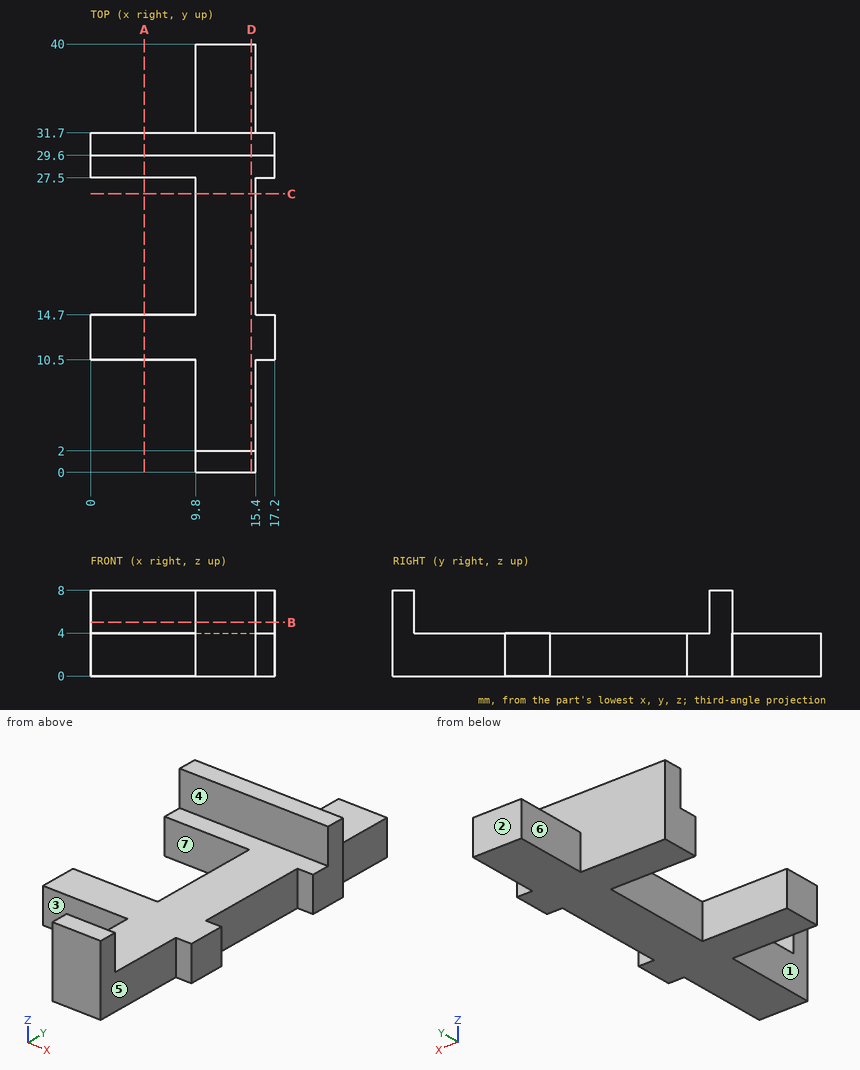
Study the drawing (mm; zero at the part's minimum x, y, z) and answer. A direction names the side the tool comes from. Give positions to 0.01 mm unless a question says otherwise; leave off trailing zeros. Order: outer loops, then holes, each group sorted by start corner. A loop starts at its lowest first (then second) coordinate and runs counter-clockwise, first axis right, second up. Notation, with made-up numbers: (82.25, -28.75) - (107.25, -28.75) arc R11 ccw to (107.25, -18.75) - close; hole circle Ø5 at (73.25, 17). An arc over 180 degrees is marked (long way). Use one line per item in the form item = value. Start each with the question number.
(1) Consider line 1 (Y direction, x = 10, z = 7.75); line 2 (Y direction, x = 4.75, z = 1.5); line 3 (Y direction, x = 9, z = 5.75). Determine where each line is inside the solid, lowest interval first. Write a range as from..to.
(2) A cutting plane is placed at B-B, the plane z = 5. Write down the section's boundary in (x, y).
(3) A cutting plane is placed at C-C, the plane y = 26. Write down the section's boundary in (x, z), then the cut area to 3 significant figures.
(4) A cutting plane is placed at D-D, the plane x = 15. Write down the section's boundary in (y, z).
(5) A cutting plane is placed at A-A, the plane x = 5. Write down the section's boundary in (y, z).
(6) Flat-ended cylindrical pins translate along their axes: pin 1 Ø1 at (y, z) = (22, 2.5) entering from -X; pin 2 Ø4.5 at (x, z) = (4.5, 1) entering from -Y; pin 3 Ø1.5 at (x, y) = (15, 19.5) entering from +Z. Find the tip coordinate at first contact, or state that the pin passes through.
(7) For the marked faces 5, 6 and 7, determine the directions among +Z, -Z, +X, -X, +Y, -Y from which every point of the face is accessible in a straight line to the end or side of a thin tool.
(8) The mould has two halves that part along Y. Classify the marked faces 1, 2, 3 and 4: released by +Y, released by -Y, zero draft, split by the parting line, or undercut.
Ans:
q1.line_1 = 0..2, 29.6..31.7
q1.line_2 = 10.5..14.7, 27.5..31.7
q1.line_3 = 29.6..31.7
q2.outline = (0, 29.6) - (17.2, 29.6) - (17.2, 31.7) - (0, 31.7) - close; (9.8, 0) - (15.4, 0) - (15.4, 2) - (9.8, 2) - close
q3.outline = (9.8, 0) - (15.4, 0) - (15.4, 4) - (9.8, 4) - close
q3.area = 22.4 mm^2
q4.outline = (0, 0) - (40, 0) - (40, 4) - (31.7, 4) - (31.7, 8) - (29.6, 8) - (29.6, 4) - (2, 4) - (2, 8) - (0, 8) - close
q5.outline = (10.5, 0) - (14.7, 0) - (14.7, 4) - (10.5, 4) - close; (27.5, 0) - (31.7, 0) - (31.7, 8) - (29.6, 8) - (29.6, 4) - (27.5, 4) - close
q6.pin_1 = 9.8
q6.pin_2 = 10.5
q6.pin_3 = 4
q7.face_5 = +Z, -Z, +X, -Y
q7.face_6 = +Z, -Z, -X, +Y
q7.face_7 = +Z, -Z, -X
q8.face_1 = zero draft
q8.face_2 = released by +Y
q8.face_3 = released by -Y
q8.face_4 = undercut
